Part print with two shaded views. Sizes in mm from the minimum x, y, z corner. A direction names the side the tool comes from. Round coordinates to 2 decimals unless told otherwise and drop trailing zeros. Loops run counter-clockwise (first coordinate to the right, second up) from the corner with the lowest first, then second, coordinate; pieces in that order, holes last. Notation, with made-up numbers: M 89,7 L 127,7 A35 cw 127,44 Z; hole C 14.5,-27 d4. An arc over 180 degrees is marked long. Use a Markdown table: item, result. Add a question column.
Item 1: Pin check, flat tips, straight feed: P1, Ø3, axis at y = 20, z = 36.5, coming from the +X side; P2, Ø4, axis at y = 4.5, z = 34, coming from the -X side; P3, Ø2, axis at y = 9.5, z = 37, coming from the -X side. Stop position of each tip, or through.
Item 2: Wall check: L1, parallel to X at y = 13, z = 33; L2, parallel to Z at x = 2.5, y = 10.5; L3, parallel to Y at x = 20.25, z = 9.5. Give the ranges that are in metal, low to high. Write a range as from..to.
Item 3: Saw through at A-A on y = 12.5. Write the cut outline in (x, z), then the cut area to 3 significant figures.
Item 4: Saw through at C-C on z = 27. Write the cut outline in (x, y).
Item 5: Tool access for the marked faces 1 and 2: list every direction of +Z, -Z, +X, -X, +Y, -Y with a clear straight run to the whole face (end or side of a thin tool).
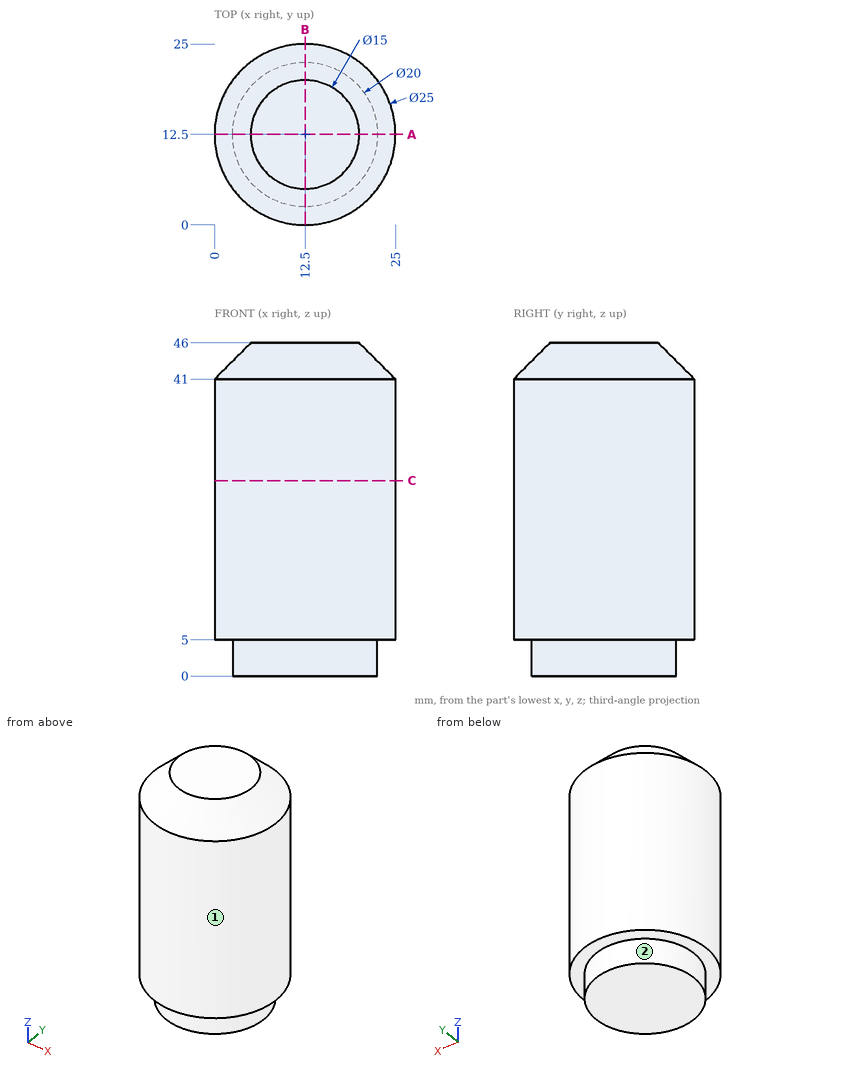
Entries:
| question | item | result |
|---|---|---|
| 1 | P1 | x = 23.47 |
| 1 | P2 | x = 1.53 |
| 1 | P3 | x = 0.16 |
| 2 | L1 | 0.01..24.99 |
| 2 | L2 | 5..43.3 |
| 2 | L3 | 2.69..22.31 |
| 3 | outline | M 0,5 L 2.5,5 L 2.5,0 L 22.5,0 L 22.5,5 L 25,5 L 25,41 L 20,46 L 5,46 L 0,41 Z |
| 3 | area | 1,100 mm2 |
| 4 | outline | C 12.5,12.5 d25 |
| 5 | face 1 | +Z, -Z |
| 5 | face 2 | -Z |
